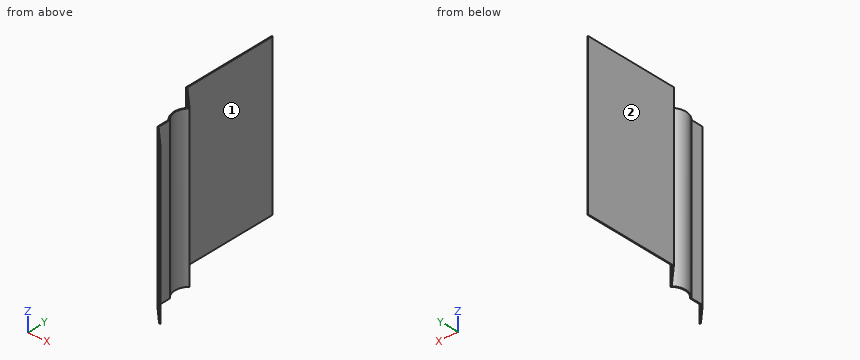
Autodesk Inventor part; units mm, degrees
ref_plane "YZ Plane" through (0, 0, 0) normal (1, 0, 0) x (0, 1, 0)
ref_plane "XZ Plane" through (0, 0, 0) normal (0, 1, 0) x (-1, 0, 0)
ref_plane "XY Plane" through (0, 0, 0) normal (0, 0, 1) x (1, 0, 0)
sketch "Sketch1" plane through (0, 0, 0) normal (0, 0, 1) x (1, 0, 0)
  circle A0 centre (-0.0003, -247.8) radius 2.5
  line L0 (-100, -150) -> (-36.4384, -213.5616)
  line L1 (-100, -150) -> (-50, -150) construction
  line L2 (-36.4384, -213.5616) -> (-36.4394, -213.5606)
  line L3 (-35.3556, -283.1553) -> (-35.3556, -323.1553)
  line L4 (-35.3556, -283.1553) -> (4.6444, -283.1553) construction
  line L5 (-35.3556, -323.1553) -> (21.2129, -379.7239)
  arc A1 (-36.4384, -213.5616) -> (-35.3556, -283.1553) centre (-0.0003, -247.8) ccw
  line L6 (-32.3556, -281.8901) -> (-32.3556, -321.9127)
  line L7 (-32.3556, -321.9127) -> (25.4556, -379.7239)
  line L8 (-97, -148.7574) -> (-32.1971, -213.5602)
  arc A2 (-32.1971, -213.5602) -> (-32.3556, -281.8901) centre (-0.0003, -247.8) ccw
  line L9 (21.2129, -379.7239) -> (25.4556, -379.7239)
  line L10 (-100, -150) -> (-100, 150)
  line L11 (-97, -148.7574) -> (-97, 150)
  line L12 (-100, 150) -> (-97, 150)
  dimension "d0" = 5
  dimension "d1" = 45
  dimension "d3" = 50
  dimension "d5" = 40
  dimension "d6" = 90
  dimension "d7" = 80
  dimension "d8" = 135
  dimension "d13" = 3
  dimension "d16" = 3
  dimension "d17" = 3
  dimension "d19" = 35.3553
  dimension "d20" = 3
  dimension "d21" = 300
extrude "Extrusion1" add sketch "Sketch1" against normal blind 494 contours L10 L12 L11 L8 A2 L6 L7 L9 L5 L3 A1 L0
properties part number "back"
For this review, take the finished solid that the model builds, in its own axes (mm). Face numbers are marked on the shaded views. A direction names the side the tool comes from. Round coordinates to 2 decimals unless told otherwise and drop trailing zeros. Write each loop counter-clockwise with the first axis right and the second up, starting at its lowest first coordinate (ties: lowest second). Pieces come first, ordered by that corner, then holes.
1) Machinability: for the marked faces 1 and 2, which of the approach directions +Z, -Z, +X, -X, +Y, -Y give a long, thin tool a straight path to every point of the face, cutting with its end or side? Answer none if there is none.
Answer below:
face 1: +Z, -Z, +X, +Y
face 2: +Z, -Z, -X, +Y, -Y
2) Insertion check: pin 1 Ø1 at (y, z) = (-178, -185) entering from -X; pin 2 Ø12 at (y, z) = (-307.5, -250.5) entering from +X; pin 3 Ø12 at (x, z) = (-86, -426.5) entering from +Y. Each pin has a flat end and moves straight along its axis. Give the tip position at first contact, or say it passes through.
Answer below:
pin 1: stops at x = -72.5
pin 2: stops at x = -32.36
pin 3: stops at y = -153.76
3) Take a section at A-A on z = -415. Give the boundary of the cut face in (x, y).
Answer below:
outline: (-100, -150) - (-36.44, -213.56) arc R50 ccw to (-35.36, -283.16) - (-35.36, -323.16) - (21.21, -379.72) - (25.46, -379.72) - (-32.36, -321.91) - (-32.36, -281.89) arc R47 cw to (-32.2, -213.56) - (-97, -148.76) - (-97, 150) - (-100, 150) - close
4) Take a section at B-B on y = -114.5. Give the boundary of the cut face in (x, z).
Answer below:
outline: (-100, -494) - (-97, -494) - (-97, 0) - (-100, 0) - close
5) Take a section at C-C on x = -12.5. Give the boundary of the cut face in (y, z), then the cut area to 3 significant figures.
Answer below:
outline: (-346.01, -494) - (-341.77, -494) - (-341.77, 0) - (-346.01, 0) - close
area: 2,100 mm2
6) For line 1 along X through (y, z) = (83, -457); line 2 along Y through (x, z) = (-34.5, -200.5); line 3 along X through (y, z) = (-311.5, -325.5), list the stretches that pass through material, from the lowest coordinate up.
Answer below:
line 1: x = -100 to -97
line 2: y = -324.01 to -279.72, -215.88 to -211.26
line 3: x = -35.36 to -32.36
